```python
from build123d import *

# Parameters (mm, degrees)
BOSS_EXTRU_1_DEPTH      = 46
CONG_1_R                = 2
ESQUISSE2_W             = 36
ESQUISSE2_H             = 20
BOSS_EXTRU_2_DEPTH      = 4
CONG_3_R                = 1
ESQUISSE4_R             = 6.5
BOSS_EXTRU_3_DEPTH      = 10
ESQUISSE5_R             = 5
ESQUISSE5_R_2           = 3
ENL_V_MAT_EXTRU_1_DEPTH = 2
BOSS_EXTRU_4_DEPTH      = 4


with BuildPart() as part:
    # Esquisse1 → Boss.-Extru.1 (new body)
    with BuildSketch(Plane.XY):
        Polygon((0, -13.5), (28.5, -13.5), (28.5, 13.5), (-28.5, 13.5), (-28.5, -13.5), align=None)
    extrude(amount=BOSS_EXTRU_1_DEPTH)

    # Congé1
    cong_1_edges = [part.edges().sort_by_distance(p)[0] for p in [
        (-28.5, -13.5, 23),
        (-28.5, 13.5, 23),
        (28.5, 13.5, 23),
        (28.5, -13.5, 23),
    ]]
    fillet(cong_1_edges, radius=CONG_1_R)

    # Esquisse2 → Boss.-Extru.2 (add)
    with BuildSketch(Plane(origin=(0, 0, 0), x_dir=(-1, 0, 0), z_dir=(0, 0, -1))):
        with Locations((6, 0)):
            Rectangle(ESQUISSE2_W, ESQUISSE2_H)
    extrude(amount=BOSS_EXTRU_2_DEPTH)

    # Congé3
    cong_3_edges = [part.edges().sort_by_distance(p)[0] for p in [
        (-24, 10, -2),
        (12, 10, -2),
        (12, -10, -2),
        (-24, -10, -2),
    ]]
    fillet(cong_3_edges, radius=CONG_3_R)

    # Esquisse4 → Boss.-Extru.3 (add)
    with BuildSketch(Plane(origin=(0, 0, -4), x_dir=(-1, 0, 0), z_dir=(0, 0, -1))):
        with Locations(Location((11.5, 0, 0), (0, 0, 180))):
            Circle(ESQUISSE4_R)
    extrude(amount=BOSS_EXTRU_3_DEPTH)

    # Esquisse5 → Enlèv. mat.-Extru.1 (cut)
    with BuildSketch(Plane(origin=(0, 0, -14), x_dir=(-1, 0, 0), z_dir=(0, 0, -1))):
        with Locations((11.5, 0)):
            Circle(ESQUISSE5_R)
        with Locations((11.5, 0)):
            Circle(ESQUISSE5_R_2, mode=Mode.SUBTRACT)
    extrude(amount=-ENL_V_MAT_EXTRU_1_DEPTH, mode=Mode.SUBTRACT)

    # Esquisse7 → Boss.-Extru.4 (add)
    with BuildSketch(Plane(origin=(0, 0, 0), x_dir=(-1, 0, 0), z_dir=(0, 0, -1))):
        with BuildLine():
            Line((-12, -5), (-12, 0))
            Line((-12, 0), (-12, 5))
            ThreePointArc((-12, 5), (-17, 0), (-12, -5))
        make_face()
    extrude(amount=BOSS_EXTRU_4_DEPTH)


solid = part.part
```
Model file for the job. Use its own axes, mm. A direction names the side the tool comes from. Round coordinates to 2 decimals unless told otherwise and drop trailing zeros. Loops run counter-clockwise (first coordinate to the right, second up) from the corner with the lowest first, then second, coordinate; pieces in that order, holes last. Notation, with made-up numbers: M 0.25,82.5 L 18.25,82.5 A7 cw 18.25,88.5 Z; hole C 71,30.5 d7. An arc over 180 degrees is marked long. Put each result on its own line as item: value. Start each with the question number.
Item 1: 3-axis set-ups, long thin cutter, end or side, ignore diameter. For faces 4 (the face through (17, 0, -2)), 5 (the face through (-14, -2, -12)), 6 (the face through (12, -7, -2)): which of +Z, -Z, +X, -X, +Y, -Y reach the whole face in a straight line?
Item 2: Mould opens along Y. For faces 1 (the face through (12, 7, -2)), 2 (the face through (-16.27, 1.5, -13.01)), 3 (the face through (-6, 10, -2)) say: released by +Y, released by -Y, zero draft, split by the parting line, or undercut.
Item 3: Drop flat-ended pins along their axis: P1, Ø2, axis at y = 0.5, z = -2.5, coming from the -X side; P2, Ø2, axis at x = 0, z = -2.5, coming from the -Y side; P3, Ø3, axis at y = -8, z = -2.5, coming from the +X side. Give the stop position or say it passes through.
Item 4: Cut at D-D (x = 14.5). List the corners of the cut face in (y, z).
Item 5: Cut at A-A (x = -11.5). List the corners of the cut face in (y, z), then the cut area to 3 significant figures.
Item 6: Cut at C-C (y = 10.75). List the corners of the cut face in (x, z).
Item 7: Drill centre lines: line 1 along Y through (x, z) = (-11.5, -12.65); line 2 along X through (y, z) = (-11.75, 42); line 3 along Z through (x, y) = (-15.5, 9.5). Where is each one in solid material? Low to high.
Item 8: Cut at B-B (y = 0). List the corners of the cut face in (x, z), then the cut area to 3 significant figures.
Answer block:
1. face 4: -Z, +X
1. face 5: -Z
1. face 6: -Z, +X, -Y
2. face 1: zero draft
2. face 2: undercut
2. face 3: released by +Y
3. P1: x = -24
3. P2: y = -10
3. P3: x = 12
4. outline: M -13.5,0 L -4.33,0 L -4.33,-4 L 4.33,-4 L 4.33,0 L 13.5,0 L 13.5,46 L -13.5,46 Z
5. outline: M -13.5,0 L -10,0 L -10,-4 L -6.5,-4 L -6.5,-14 L -5,-14 L -5,-12 L -3,-12 L -3,-14 L 3,-14 L 3,-12 L 5,-12 L 5,-14 L 6.5,-14 L 6.5,-4 L 10,-4 L 10,0 L 13.5,0 L 13.5,46 L -13.5,46 Z
5. area: 1,440 mm2
6. outline: M -28.5,0 L 28.5,0 L 28.5,46 L -28.5,46 Z
7. line 1: -6.5 to -5, -3 to 3, 5 to 6.5
7. line 2: -28.48 to 28.48
7. line 3: -4 to 46
8. outline: M -28.5,0 L -24,0 L -24,-4 L -18,-4 L -18,-14 L -16.5,-14 L -16.5,-12 L -14.5,-12 L -14.5,-14 L -8.5,-14 L -8.5,-12 L -6.5,-12 L -6.5,-14 L -5,-14 L -5,-4 L 17,-4 L 17,0 L 28.5,0 L 28.5,46 L -28.5,46 Z
8. area: 2,910 mm2
